Autodesk Inventor part; units mm, degrees
ref_plane "Work Plane1" through (-20.8209, 0, 0) normal (0, -0.866, -0.5) x (1, 0, 0)
ref_plane "YZ Plane" through (0, 0, 0) normal (1, 0, 0) x (0, 1, 0)
ref_plane "XZ Plane" through (0, 0, 0) normal (0, 1, 0) x (-1, 0, 0)
sketch "Sketch1" plane through (0, 0, 0) normal (1, 0, 0) x (0, 1, 0)
  line L0 (-10.9697, 0) -> (-5.4848, 9.5)
  line L1 (-5.4848, 9.5) -> (5.4848, 9.5)
  line L2 (5.4848, 9.5) -> (10.9697, 0)
  line L3 (10.9697, 0) -> (5.4848, -9.5)
  line L4 (5.4848, -9.5) -> (-5.4848, -9.5)
  line L5 (-5.4848, -9.5) -> (-10.9697, 0)
  point P0 (0, 0)
  point P1 (0, 0)
  dimension "d0" = 21.9393
extrude "Body" add sketch "Sketch1" along normal blind 10
sketch "Sketch2" plane through (0, 0, 0) normal (0, 0, 1) x (1, 0, 0)
  line L0 (0, 5.4848) -> (0, 10.9697)
  line L1 (0, 10.9697) -> (10, 10.9697)
  line L2 (10, 5.4848) -> (10, 10.9697)
  line L3 (-2, 0) -> (12, 0)
  line L4 (1.397, 10.9697) -> (0, 8.55)
  line L5 (8.603, 10.9697) -> (10, 8.55)
  dimension "d3" = 30
  dimension "d4" = 30
  dimension "d5" = 17.1
  dimension "d6" = 17.1
revolve "Chamfer1" cut sketch "Sketch2" angle 360 about axis through (-10, 0, 0) along (1, 0, 0)
sketch "Sketch3" plane through (10, 0, 0) normal (1, 0, 0) x (0, 0, -1)
  arc A0 (-0.625, -1.0825) -> (0.625, -1.0825) centre (0, 0) ccw
hole "Thread" at (10, 0, 0) direction (-1, 0, 0) diameter 10.106 end through all
chamfer "Chamfer2" distance 0.9472 angle 30 1 edges at (10, 0, 5.053) measured on face at (10, 7.2892, -0.8851)
chamfer "Chamfer3" distance 0.9472 angle 30 1 edges at (0, 0, 5.053) measured on face at (0, 7.2892, -0.8851)
ref_plane "Work Plane1" through (-20.8209, 0, 0) normal (0, -0.866, -0.5) x (1, 0, 0)
equation "\"d0\" = 1.1547 * SW"
equation "\"d1\" = KOH"
equation "\"d8\" = -0.5 * GD1 + 0.5 * NND"
equation "\"d40\" = -0.5 * GD1 + 0.5 * NND"
equation "\"d10\" = -0.5 * GD1 + 0.5 * NND"
equation "\"d41\" = -0.5 * GD1 + 0.5 * NND"
equation "\"d3\" = ANG1"
equation "\"d4\" = ANG2"
equation "\"d5\" = SW0"
equation "\"d6\" = SW01"
equation "\"ANG1\" = 30deg"
equation "\"ANG2\" = 30deg"
equation "\"NND\" = 12"
equation "\"KOH\" = 10"
equation "\"SW\" = 19"
equation "\"SW0\" = 17.1"
equation "\"SW01\" = SW0"
equation "\"GUL\" = 0.541266 * PTC"
equation "\"LADI\" = 18.05"
equation "\"TOA\" = 30deg"
equation "\"FAWI\" = 30deg"
equation "\"PTC\" = 1.75"
equation "\"THREADDIA\" = 12"
equation "\"E0\" = 1.155 * SW"
equation "\"GAL\" = 0.541266 * PTC"
properties part number "Nut M12-6H GOST 5915-70" material "Steel"
Geometry check sheet. Reference: the model listing, model coordinates, mm. Give positions to 0.01 mm unless a question says otherwise; leave off trailing zeros. Loops run counter-clockwise (first coordinate to the right, second up) from the corner with the lowest first, then second, coordinate; pieces in that order, holes last. Notation, with made-up numbers: M 36,30.25 L 41,30.25 A10 cw 41,35.25 Z; hole C 87.5,60.5 d8. An arc over 180 degrees is marked long. Answer as a JSON object with one key per item and string values. Group by question number.
Item 1: Gauge pin test, flat ends, axial feed: pin 1 (1.5 mm diameter, centred on x = 1.5, z = -7, fed in from +Y); pin 2 (5 mm diameter, centred on x = 4, y = 7, fed in from +Z); pin 3 (1.5 mm diameter, centred on x = 7, z = -3, fed in from +Y); pin 4 (1 mm diameter, centred on x = 4, z = -2.5, fed in from -Y) (3 decimals). Record the tip position at first contact, or that the pin passes through.
Item 2: Sectioned sample at B-B on x = 6. Record the boundary of the cut face in (y, z).
Item 3: Sectioned sample at A-A on y = 0. Record the boundary of the cut face in (x, z), plus the area to 3 significant figures.
Item 4: Material ranges on L1, parallel to Z at x = 5, y = 0; L2, parallel to Z at x = 6.75, y = -2.75; L3, parallel to Y at x = 6.5, z = -1, recorded low to high.
Item 5: Mould release check, pull along Z, two halves, no side actions. Record for faces 1 (the flat face through (0, 2, 6)), 2 (the flat face through (4.938, 8.266, -4.683)), 3 (the cylindrical face through (4.938, 3.075, 4.01)): pulls with the +Z half, pulls with the -Z half, needs draft (parallel to the pull), parting line crosses it, or undercut.
Item 6: Sectioned sample at C-C on x = 9. Record the boundary of the cut face in (y, z).
Findings below:
{
 "1": {"pin 1": "y = 7.36", "pin 2": "z = 9.5", "pin 3": "y = 9.67", "pin 4": "y = -9.815"},
 "2": {"outline": "M -10.97,0 L -5.48,-9.5 L 5.48,-9.5 L 10.97,0 L 5.48,9.5 L -5.48,9.5 Z; hole C 0,0 d10.11"},
 "3": {"outline": "M 0,-8.55 L 0.55,-9.5 L 9.45,-9.5 L 10,-8.55 L 10,-6 L 9.45,-5.05 L 0.55,-5.05 L 0,-6 Z; M 0,6 L 0.55,5.05 L 9.45,5.05 L 10,6 L 10,8.55 L 9.45,9.5 L 0.55,9.5 L 0,8.55 Z", "area": "86.9 mm2"},
 "4": {"L1": "-9.5 to -5.05, 5.05 to 9.5", "L2": "-9.5 to -4.24, 4.24 to 9.5", "L3": "-10.39 to -4.95, 4.95 to 10.39"},
 "5": {"face 1": "needs draft", "face 2": "pulls with the -Z half", "face 3": "undercut"},
 "6": {"outline": "M -10.19,-1.34 L -6.26,-8.16 A10.28 ccw -3.93,-9.5 L 3.93,-9.5 A10.28 ccw 6.26,-8.16 L 10.19,-1.34 A10.28 ccw 10.19,1.34 L 6.26,8.16 A10.28 ccw 3.93,9.5 L -3.93,9.5 A10.28 ccw -6.26,8.16 L -10.19,1.34 A10.28 ccw Z; hole C 0,0 d10.11"}
}
